Autodesk Inventor part; units mm, degrees
ref_plane "YZ Plane" through (0, 0, 0) normal (1, 0, 0) x (0, 1, 0)
ref_plane "XZ Plane" through (0, 0, 0) normal (0, 1, 0) x (-1, 0, 0)
ref_plane "XY Plane" through (0, 0, 0) normal (0, 0, 1) x (1, 0, 0)
sketch "Sketch1" plane through (0, 0, 0) normal (0, 0, 1) x (1, 0, 0)
  line L0 (0, 0) -> (190.5, 0)
  line L1 (190.5, 0) -> (190.5, 25.4)
  line L2 (190.5, 25.4) -> (0, 25.4)
  line L3 (0, 25.4) -> (0, 0)
  dimension "d0" = 190.5
  dimension "d1" = 25.4
extrude "Extrusion1" add sketch "Sketch1" along normal blind 50.8
shell "Shell1" thickness 3.175 removed faces 2 at (0, 16.9333, 33.8667) at (190.5, 8.4667, 16.9333)
sketch "Sketch4" plane through (0, 0, 0) normal (0, 0, -1) x (-1, 0, 0)
  line L0 (0, 25.4) -> (0, 0)
  line L1 (-190.5, 25.4) -> (0, 25.4)
  line L2 (-190.5, 0) -> (-190.5, 25.4)
  circle A0 centre (-139.7, 12.7) radius 3.175
  circle A1 centre (-50.8, 12.7) radius 3.175
  dimension "d5" = 50.8
  dimension "d6" = 50.8
  dimension "d7" = 12.7
  dimension "d8" = 12.7
  dimension "d9" = 6.35
extrude "Extrusion2" cut sketch "Sketch4" against normal through all
sketch "Sketch5" plane through (0, 0, 50.8) normal (0, 0, 1) x (1, 0, 0)
  circle A0 centre (50.8, 12.7) radius 3.175
  circle A1 centre (139.7, 12.7) radius 3.175
  circle A2 centre (50.8, 12.7) radius 6.35
  circle A3 centre (139.7, 12.7) radius 6.35
  dimension "d12" = 12.7
  dimension "d13" = 12.7
extrude "Extrusion3" cut sketch "Sketch5" against normal up to next
properties part number "SpatulaPivotMount" material "Aluminum-6061"
Source: CAD feature listing. Evaluate the final solid. Frame: model axes, mm. A direction names the side the tool comes from. Give positions to 0.01 mm unless a question says otherwise; leave off trailing zeros. Loops run counter-clockwise (first coordinate to the right, second up) from the corner with the lowest first, then second, coordinate; pieces in that order, holes last. Notation, with made-up numbers: (11, -11) -> (34, -11) arc R14 cw to (34, 13) -> close; hole circle Ø10 at (-28.75, 36). An arc over 180 degrees is marked (long way). Put each result on its own line as item: value. Start each with the question number.
1) Cut plane C-C (y = 12.7). Return loops of the section in (x, z) (3 decimals).
2) Cut plane A-A (z = 14.5). Return loops of the section in (x, y) (3 decimals).
3) Reachability of faces 5 (the face through (53.97, 12.84, 1.57)), 6 (the face through (94, 13, 47.625)), 7 (the face through (56.857, 14.607, 49.235)) from +Z, -Z, +X, -X, +Y, -Y: full face, straight path, thin tool, end or side. Return the list, or none.
4) Draft query along Y for faces 1 (the face through (97, 22.225, 25)), 2 (the face through (0, 23, 27)), 3 (the face through (136.77, 11.48, 1.57)), 4 (the face through (94, 0, 25)). Return one class per face: released by +Y, released by -Y, zero draft, split by the parting line, or undercut.
5) Cut plane D-D (x = 139.7). Return loops of the section in (y, z) (3 decimals), then the cut area to 3 significant figures.
6) Material intervals for probe 1 along Z at (x, y) = (174.5, 9.5) (3 decimals); probe 2 along Y at (x, z) = (50.8, 49.5); probe 3 along Y at (x, z) = (78, 34.5) (3 decimals), sorted ascending.
7) Contact query for a flat-ended pin moving along its axis: P1, Ø10, axis at x = 139.7, y = 12.7, coming from the +Z side (3 decimals). Output: stop coordinate, or through.
8) Cut plane B-B (x = 94.5). Return loops of the section in (y, z) (3 decimals).
Results are:
1. outline: (0, 0) -> (47.625, 0) -> (47.625, 3.175) -> (0, 3.175) -> close; (0, 47.625) -> (44.45, 47.625) -> (44.45, 50.8) -> (0, 50.8) -> close; (53.975, 0) -> (136.525, 0) -> (136.525, 3.175) -> (53.975, 3.175) -> close; (57.15, 47.625) -> (133.35, 47.625) -> (133.35, 50.8) -> (57.15, 50.8) -> close; (142.875, 0) -> (190.5, 0) -> (190.5, 3.175) -> (142.875, 3.175) -> close; (146.05, 47.625) -> (190.5, 47.625) -> (190.5, 50.8) -> (146.05, 50.8) -> close
2. outline: (0, 0) -> (190.5, 0) -> (190.5, 3.175) -> (0, 3.175) -> close; (0, 22.225) -> (190.5, 22.225) -> (190.5, 25.4) -> (0, 25.4) -> close
3. face 5: +Z, -Z
3. face 6: +X, -X
3. face 7: +Z
4. face 1: undercut
4. face 2: zero draft
4. face 3: undercut
4. face 4: released by -Y
5. outline: (0, 0) -> (9.525, 0) -> (9.525, 3.175) -> (3.175, 3.175) -> (3.175, 47.625) -> (6.35, 47.625) -> (6.35, 50.8) -> (0, 50.8) -> close; (15.875, 0) -> (25.4, 0) -> (25.4, 50.8) -> (19.05, 50.8) -> (19.05, 47.625) -> (22.225, 47.625) -> (22.225, 3.175) -> (15.875, 3.175) -> close
5. area: 383 mm2
6. probe 1: z = 0 to 3.175, 47.625 to 50.8
6. probe 2: y = 0 to 6.35, 19.05 to 25.4
6. probe 3: y = 0 to 3.175, 22.225 to 25.4
7. P1: stops at z = 3.175
8. outline: (0, 0) -> (25.4, 0) -> (25.4, 50.8) -> (0, 50.8) -> close; hole (3.175, 3.175) -> (22.225, 3.175) -> (22.225, 47.625) -> (3.175, 47.625) -> close
